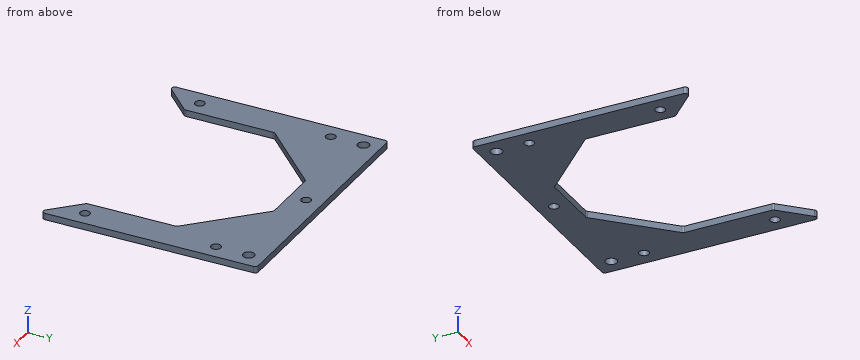
from build123d import *

# Parameters (mm, degrees)
SKETCH_R   = 3.5
SKETCH_R_2 = 3
PAD_DEPTH  = 4


with BuildPart() as part:
    # Sketch → Pad (new body)
    with BuildSketch(Plane.XY):
        with BuildLine():
            Line((-78, 8), (-78, -119.313708))
            ThreePointArc((-78, -119.313708), (-76.765367, -121.161468), (-74.585786, -120.727922))
            Line((-74.585786, -120.727922), (-58.585786, -104.727922))
            ThreePointArc((-58.585786, -104.727922), (-58.152241, -104.079075), (-58, -103.313708))
            Line((-58, -50), (-58, -103.313708))
            ThreePointArc((-57.414214, -48.585786), (-57.847759, -49.234633), (-58, -50))
            Line((-57.414214, -48.585786), (-19.414214, -10.585786))
            ThreePointArc((-18, -10), (-18.765367, -10.152241), (-19.414214, -10.585786))
            Line((-18, -10), (18, -10))
            ThreePointArc((19.414214, -10.585786), (18.765367, -10.152241), (18, -10))
            Line((19.414214, -10.585786), (57.414214, -48.585786))
            ThreePointArc((58, -50), (57.847759, -49.234633), (57.414214, -48.585786))
            Line((58, -50), (58, -103.313708))
            ThreePointArc((58, -103.313708), (58.152241, -104.079075), (58.585786, -104.727922))
            Line((58.585786, -104.727922), (74.585786, -120.727922))
            ThreePointArc((74.585786, -120.727922), (76.765367, -121.161468), (78, -119.313708))
            Line((78, -119.313708), (78, 8))
            ThreePointArc((78, 8), (77.414214, 9.414214), (76, 10))
            Line((76, 10), (-76, 10))
            ThreePointArc((-76, 10), (-77.414214, 9.414214), (-78, 8))
        make_face()
        with Locations((-68, 0)):
            Circle(SKETCH_R, mode=Mode.SUBTRACT)
        with Locations((68, 0)):
            Circle(SKETCH_R, mode=Mode.SUBTRACT)
        with Locations((-68, -20)):
            Circle(SKETCH_R_2, mode=Mode.SUBTRACT)
        with Locations((-68, -100)):
            Circle(SKETCH_R_2, mode=Mode.SUBTRACT)
        with Locations((68, -20)):
            Circle(SKETCH_R_2, mode=Mode.SUBTRACT)
        with Locations((68, -100)):
            Circle(SKETCH_R_2, mode=Mode.SUBTRACT)
        Circle(SKETCH_R_2, mode=Mode.SUBTRACT)
    extrude(amount=PAD_DEPTH)


solid = part.part
Geometry check sheet. Reference: the model listing, model coordinates, mm. Give positions to 0.01 mm unless a question says otherwise; leave off trailing zeros. Order: outer loops, then holes, each group sorted by start corner. A loop starts at its lowest first (then second) coordinate and runs counter-clockwise, first axis right, second up.
1. Scan lines: line 1 (X direction, y = -78.5, z = 0.55); line 2 (X direction, y = -98.5, z = 0.8); line 3 (Y direction, x = 0, z = 2.8). Record each from-to range of solid material in increasing order.
Completed:
line 1: x = -78 to -58, 58 to 78
line 2: x = -78 to -70.6, -65.4 to -58, 58 to 65.4, 70.6 to 78
line 3: y = -10 to -3, 3 to 10
2. Depth check by flat-ended pin: pin 1 (1 mm diameter, centred on x = 37.5, z = 2.5, fed in from -Y); pin 2 (1.2 mm diameter, centred on x = -0.5, z = 2, fed in from -Y); pin 3 (6.5 mm diameter, centred on x = 68, y = 0, fed in from -Z). Enter the tip coordinate at first touch or a pass-through.
Completed:
pin 1: stops at y = -29.17
pin 2: stops at y = -10
pin 3: passes through
3. Sectioned sample at C-C (z = 2.35). Record the boundary of the cut face in (x, y).
Completed:
outline: (-78, -119.31) arc R2 ccw to (-74.59, -120.73) - (-58.59, -104.73) arc R2 ccw to (-58, -103.31) - (-58, -50) arc R2 cw to (-57.41, -48.59) - (-19.41, -10.59) arc R2 cw to (-18, -10) - (18, -10) arc R2 cw to (19.41, -10.59) - (57.41, -48.59) arc R2 cw to (58, -50) - (58, -103.31) arc R2 ccw to (58.59, -104.73) - (74.59, -120.73) arc R2 ccw to (78, -119.31) - (78, 8) arc R2 ccw to (76, 10) - (-76, 10) arc R2 ccw to (-78, 8) - close; hole circle Ø7 at (-68, 0); hole circle Ø6 at (-68, -100); hole circle Ø6 at (-68, -20); hole circle Ø6 at (0, 0); hole circle Ø7 at (68, 0); hole circle Ø6 at (68, -100); hole circle Ø6 at (68, -20)
4. Sectioned sample at B-B (y = -65.5). Record the boundary of the cut face in (x, z).
Completed:
outline: (-78, 0) - (-58, 0) - (-58, 4) - (-78, 4) - close; (58, 0) - (78, 0) - (78, 4) - (58, 4) - close
5. Sectioned sample at A-A (y = 0). Record the boundary of the cut face in (x, z), then the cut area to 3 significant figures.
Completed:
outline: (-78, 0) - (-71.5, 0) - (-71.5, 4) - (-78, 4) - close; (-64.5, 0) - (-3, 0) - (-3, 4) - (-64.5, 4) - close; (3, 0) - (64.5, 0) - (64.5, 4) - (3, 4) - close; (71.5, 0) - (78, 0) - (78, 4) - (71.5, 4) - close
area: 544 mm2
6. Sectioned sample at D-D (x = -68). Record the boundary of the cut face in (y, z), then the cut area to 3 significant figures.
Completed:
outline: (-114.14, 0) - (-103, 0) - (-103, 4) - (-114.14, 4) - close; (-97, 0) - (-23, 0) - (-23, 4) - (-97, 4) - close; (-17, 0) - (-3.5, 0) - (-3.5, 4) - (-17, 4) - close; (3.5, 0) - (10, 0) - (10, 4) - (3.5, 4) - close
area: 421 mm2
